Autodesk Inventor part; units mm, degrees
ref_plane "YZ Plane" through (0, 0, 0) normal (1, 0, 0) x (0, 1, 0)
ref_plane "XZ Plane" through (0, 0, 0) normal (0, 1, 0) x (-1, 0, 0)
ref_plane "XY Plane" through (0, 0, 0) normal (0, 0, 1) x (1, 0, 0)
sketch "Sketch1" plane through (0, 0, 0) normal (0, 1, 0) x (-1, 0, 0)
  line L0 (4.9, 4.9) -> (-4.9, 4.9)
  line L1 (-4.9, 4.9) -> (-4.9, -4.9)
  line L2 (-4.9, -4.9) -> (4.9, -4.9)
  line L3 (4.9, -4.9) -> (4.9, 4.9)
  point P0 (0, 0)
  dimension "d0" = 9.8
  dimension "d1" = 9.8
  dimension "d2" = 4.9
  dimension "d3" = 4.9
extrude "Extrusion1" add sketch "Sketch1" along normal blind 13.1
sketch "Sketch2" plane through (0, 0, 0) normal (0, 0, 1) x (1, 0, 0)
  line L0 (-4.9, 13.1) -> (4.9, 13.1)
  line L1 (4.9, 13.1) -> (6.5, 12.0007)
  line L2 (6.5, 12.0007) -> (6.5, 9.8)
  line L3 (6.5, 9.8) -> (4.9, 9.8)
  line L4 (4.9, 9.8) -> (4.9, 13.1)
  line L5 (4.9, 0) -> (4.9, 13.1)
  point P0 (0, 0)
  dimension "d6" = 3.3
  dimension "d7" = 1.6
extrude "Extrusion2" add sketch "Sketch2" along normal mid plane 3.6
sketch "Sketch3" plane through (0, 13.1, 0) normal (0, 1, 0) x (1, 0, 0)
  line L0 (-3.9809, -4.385) -> (-0.5456, -4.385)
  line L1 (-0.5456, -4.385) -> (-0.5456, -0.4741)
  line L2 (-0.5456, -0.4741) -> (-3.9809, -0.4741)
  line L3 (-3.9809, -0.4741) -> (-3.9809, -4.385)
  line L4 (0.8079, 0.7571) -> (4.1425, 0.7571)
  line L5 (4.1425, 0.7571) -> (4.1425, 4.5726)
  line L6 (4.1425, 4.5726) -> (0.8079, 4.5726)
  line L7 (0.8079, 4.5726) -> (0.8079, 0.7571)
  line L8 (-0.5456, 0.7571) -> (-3.9809, 0.7571)
  line L9 (-3.9809, 0.7571) -> (-3.9809, 4.5726)
  line L10 (-3.9809, 4.5726) -> (-0.5456, 4.5726)
  line L11 (-0.5456, 4.5726) -> (-0.5456, 0.7571)
  line L12 (0.8079, -4.385) -> (4.1425, -4.385)
  line L13 (4.1425, -4.385) -> (4.1425, -0.4741)
  line L14 (4.1425, -0.4741) -> (0.8079, -0.4741)
  line L15 (0.8079, -0.4741) -> (0.8079, -4.385)
  line L16 (-3.9809, 3.3862) -> (-2.7944, 4.5726)
  line L17 (-3.9809, 1.8506) -> (-2.8874, 0.7571)
  line L18 (0.8079, -3.4193) -> (1.7736, -4.385)
  line L19 (0.8079, -1.3667) -> (1.7005, -0.4741)
  point P0 (0, 0)
  dimension "d10" = 45
  dimension "d11" = 45
extrude "Extrusion3" cut sketch "Sketch3" against normal blind 10 contours L3 L2 L1 L0 | L7 L6 L5 L4 | L8 L17 L9 L16 L10 L11 | L18 L15 L19 L14 L13 L12
sketch "Sketch4" plane through (0, 0, 0) normal (0, -1, 0) x (1, 0, 0)
  circle A0 centre (3.05, 2.2) radius 0.5
  line L0 (4.9, 4.9) -> (4.9, -4.9)
  line L1 (-4.9, 4.9) -> (4.9, 4.9)
  point P0 (0, 0)
  dimension "d15" = 1
  dimension "d16" = 1.85
  dimension "d17" = 2.7
extrude "Extrusion4" add sketch "Sketch4" along normal blind 4 and the other way blind 9
pattern_linear "Rectangular Pattern1" count 2 spacing 4.2 along (0, 0, -1) count 2 spacing 5.5 along (-1, 0, 0) of "Extrusion4"
properties part number "Molex_MiniFitJR_4Pos"
Here's how the part is built. I have some questions about the finished solid (model axes, mm). A direction names the side the tool comes from. Coordinates: 2 decimals unless noted, no trailing zeros. Order: outer loops, then holes, each group sorted by start corner. A loop starts at its lowest first (then second) coordinate and runs counter-clockwise, first axis right, second up.
Item 1: For P1, Ø1, axis at x = -2.5, z = 2.5, coming from the +Y side; P2, Ø4, axis at y = 3, z = 2.5, coming from the +X side; P3, Ø1.5, axis at x = -0.5, z = 3, coming from the -Y side, each with a flat end and sliding along its axis, tell me the tip position at first contact or that it passes through.
Result sheet:
P1: stops at y = 9
P2: stops at x = 4.9
P3: stops at y = 0
Item 2: If we section it at D-D on y = -1.75: List the corners of the cut face in (x, z) for me.
Result sheet:
outline: circle Ø1 at (-2.45, -2); circle Ø1 at (-2.45, 2.2); circle Ø1 at (3.05, -2); circle Ø1 at (3.05, 2.2)
Item 3: I need wall thicknesses on line 1 (Z direction, x = 4, y = 6.5) (3 decimals); line 2 (X direction, y = 9.5, z = 3); line 3 (Y direction, x = 2.75, z = 0). Which ranges of each line are inside material? Lowest first, please.
Result sheet:
line 1: z = -4.9 to -4.573, -0.757 to 0.474, 4.385 to 4.9
line 2: x = -4.9 to -3.98, -0.55 to 0.81, 4.14 to 4.9
line 3: y = 0 to 13.1
Item 4: If we mould it in two halves opening along X, with no side actions, what happens to faces 1 (the face through (5.689, 12.558, -0.025)), 2 (the face through (-2, 3.1, 3)), 3 (the face through (-2.5, -4, 2.2))? For each: +X half, -X half, draft (parallel to the pull), parting line (faces both ways), or undercut.
Result sheet:
face 1: +X half
face 2: undercut
face 3: draft
Item 5: If we section it at C-C on x = -2.45: List the corners of the cut face in (y, z) for me (3 decimals).
Result sheet:
outline: (-4, -2.5) - (0, -2.5) - (0, -4.9) - (13.1, -4.9) - (13.1, -4.573) - (3.1, -4.573) - (3.1, -2.5) - (9, -2.5) - (9, -1.5) - (3.1, -1.5) - (3.1, -0.757) - (13.1, -0.757) - (13.1, 0.474) - (3.1, 0.474) - (3.1, 1.7) - (9, 1.7) - (9, 2.7) - (3.1, 2.7) - (3.1, 4.385) - (13.1, 4.385) - (13.1, 4.9) - (0, 4.9) - (0, 2.7) - (-4, 2.7) - (-4, 1.7) - (0, 1.7) - (0, -1.5) - (-4, -1.5) - close
Item 6: For faces 4 (the face through (-2.5, 9, -2)), 5 (the face through (6, 9.8, 0)), 6 (the face through (-2.515, -1.972, -2.496)), 7 (the face through (6, 11, 1.8)), which set-ups out of +Z, -Z, +X, -X, +Y, -Y let a thin tool reach every point of the face, with its end or its side?
Result sheet:
face 4: +Y
face 5: +Z, -Z, +X, -Y
face 6: -Y
face 7: +Z, +X, +Y, -Y
Item 7: If we section it at B-B on z = 2.2: List the corners of the cut face in (x, y) for me.
Result sheet:
outline: (-4.9, 0) - (-2.95, 0) - (-2.95, -4) - (-1.95, -4) - (-1.95, 0) - (2.55, 0) - (2.55, -4) - (3.55, -4) - (3.55, 0) - (4.9, 0) - (4.9, 13.1) - (4.14, 13.1) - (4.14, 3.1) - (3.55, 3.1) - (3.55, 9) - (2.55, 9) - (2.55, 3.1) - (0.81, 3.1) - (0.81, 13.1) - (-0.55, 13.1) - (-0.55, 3.1) - (-1.95, 3.1) - (-1.95, 9) - (-2.95, 9) - (-2.95, 3.1) - (-3.98, 3.1) - (-3.98, 13.1) - (-4.9, 13.1) - close
Item 8: If we section it at A-A on y = 8.25: State how many separate pieces and enclosed holes the cut face has, plus the area to 3 significant figures.
Result sheet:
separate pieces: 5
enclosed holes: 4
area: 49.0 mm2
